The drawing under review shows one solid part. Ordinate dimensions are in mm from its lowest x, y, z. Coordinates: 2 decimals unless noted, no trailing zeros. Order: outer loops, then holes, each group sorted by start corner. A loop starts at its lowest first (then second) coordinate and runs counter-clockwise, first axis right, second up. Notation, with made-up numbers: (39.25, 74.25) - (52.25, 74.25) arc R18 ccw to (52.25, 92.25) - close; hole circle Ø6 at (5, 33). An arc over 180 degrees is marked (long way). Answer in a Markdown table with one row per item.
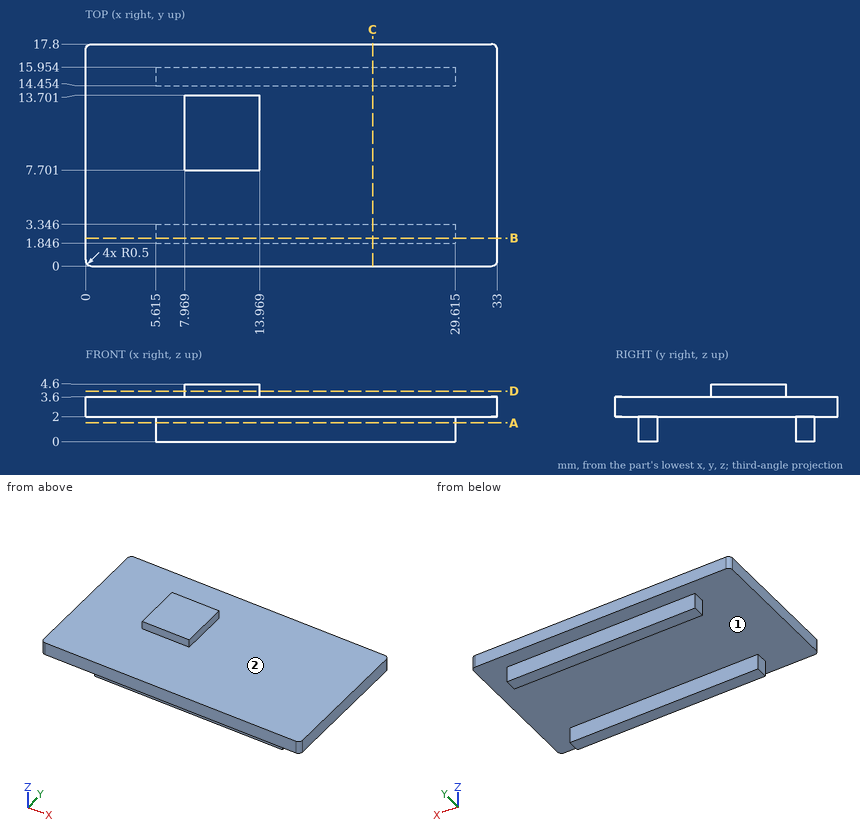
Item 1: We need section C-C, the plane x = 23. Write out the cut boundary in (y, z).
Check values:
| item | result |
|---|---|
| outline | (0, 2) - (1.85, 2) - (1.85, 0) - (3.35, 0) - (3.35, 2) - (14.45, 2) - (14.45, 0) - (15.95, 0) - (15.95, 2) - (17.8, 2) - (17.8, 3.6) - (0, 3.6) - close |
Item 2: We need section A-A, the plane z = 1.5. Write out the cut boundary in (x, y) (1 decimal).
Check values:
| item | result |
|---|---|
| outline | (5.6, 1.8) - (29.6, 1.8) - (29.6, 3.3) - (5.6, 3.3) - close; (5.6, 14.5) - (29.6, 14.5) - (29.6, 16) - (5.6, 16) - close |
Item 3: Clearance check with flat-ended pins moving along their axes: pin 1 Ø0.5 at (y, z) = (11.5, 4) entering from +X; pin 2 Ø0.5 at (y, z) = (3, 1.5) entering from +X (1 decimal); pin 3 Ø1.1 at (x, z) = (11.5, 4.5) entering from +Y. State where each tip first meets the part, or that it passes through.
Check values:
| item | result |
|---|---|
| pin 1 | x = 13.97 |
| pin 2 | x = 29.6 |
| pin 3 | y = 13.7 |
Item 4: Mouldability with a two-part tool opening along Y and no side actions: class the marked faces 1 and 2 as +Y half, -Y half, draft (parallel to the pull), parting line (faces both ways), or undercut.
Check values:
| item | result |
|---|---|
| face 1 | undercut |
| face 2 | draft |
Item 5: To check wall thickness, follow line 1 (Y direction, x = 26, z = 0.5); line 2 (Z direction, x = 16.5, y = 7); line 3 (Z direction, x = 26.5, y = 3.25). State the ranges of each line that lie inside material, in increasing order. Write a range as from..to.
Check values:
| item | result |
|---|---|
| line 1 | 1.85..3.35, 14.45..15.95 |
| line 2 | 2..3.6 |
| line 3 | 0..3.6 |
Item 6: We need section D-D, the plane z = 4.05. Write out the cut boundary in (x, y), then the cut area to 3 significant figures.
Check values:
| item | result |
|---|---|
| outline | (7.97, 7.7) - (13.97, 7.7) - (13.97, 13.7) - (7.97, 13.7) - close |
| area | 36.0 mm^2 |
Item 7: We need section B-B, the plane y = 2.25. Write out the cut boundary in (x, z) (1 decimal).
Check values:
| item | result |
|---|---|
| outline | (0, 2) - (5.6, 2) - (5.6, 0) - (29.6, 0) - (29.6, 2) - (33, 2) - (33, 3.6) - (0, 3.6) - close |
